from build123d import *

# Parameters (mm, degrees)
SKETCH_1_R          = 3.5
SKETCH_1_R_2        = 13
EXTRUDE_2_DEPTH     = 10
SKETCH_2_R          = 12.5
EXTRUDE_3_DEPTH     = 15
SKETCH_3_W          = 0.517195108
SKETCH_3_H          = 18.726193104
CUT_EXTRUDE_1_DEPTH = 26
SKETCH_4_R          = 2.5
CUT_EXTRUDE_2_DEPTH = 43.740275714


with BuildPart() as part:
    # 草图1 → 凸台-拉伸2 (new body)
    with BuildSketch(Plane.XY):
        with BuildLine():
            Line((-35, -7), (-7.740275714, -18.44147857))
            ThreePointArc((-7.740275714, -18.44147857), (0, -20), (7.740275714, -18.44147857))
            Line((7.740275714, -18.44147857), (35, -7))
            Line((35, -7), (35, 7))
            Line((35, 7), (7.740275714, 18.44147857))
            Line((7.740275714, 18.44147857), (7.740275714, 25.44147857))
            ThreePointArc((7.740275714, 25.44147857), (0, 27.494244152), (-7.740275714, 25.44147857))
            Line((-7.740275714, 25.44147857), (-7.740275714, 18.44147857))
            Line((-7.740275714, 18.44147857), (-35, 7))
            Line((-35, 7), (-35, -7))
        make_face()
        with Locations((-28, 0)):
            Circle(SKETCH_1_R, mode=Mode.SUBTRACT)
        Circle(SKETCH_1_R_2, mode=Mode.SUBTRACT)
        with Locations((28, 0)):
            Circle(SKETCH_1_R, mode=Mode.SUBTRACT)
    extrude(amount=EXTRUDE_2_DEPTH)

    # 草图2 → 凸台-拉伸3 (add)
    with BuildSketch(Plane.XY.offset(10)):
        with BuildLine():
            Line((-7.740275714, 18.44147857), (-7.740275714, 25.44147857))
            ThreePointArc((-7.740275714, 25.44147857), (0, 27.494244152), (7.740275714, 25.44147857))
            Line((7.740275714, 25.44147857), (7.740275714, 18.44147857))
            ThreePointArc((7.740275714, 18.44147857), (0, -20), (-7.740275714, 18.44147857))
        make_face()
        Circle(SKETCH_2_R, mode=Mode.SUBTRACT)
    extrude(amount=EXTRUDE_3_DEPTH)

    # 草图3 → 切除-拉伸1 (cut, through all)
    with BuildSketch(Plane.XY.offset(25)):
        with Locations((0, 21.741202931)):
            Rectangle(SKETCH_3_W, SKETCH_3_H)
    extrude(amount=-CUT_EXTRUDE_1_DEPTH, mode=Mode.SUBTRACT)

    # 草图4 → 切除-拉伸2 (cut, through all)
    with BuildSketch(Plane(origin=(7.740275714, 0, 0), x_dir=(0, 0, -1), z_dir=(1, 0, 0))):
        with Locations((-12.5, 21.086423576)):
            Circle(SKETCH_4_R)
    extrude(amount=-CUT_EXTRUDE_2_DEPTH, mode=Mode.SUBTRACT)


solid = part.part
Geometry: final body of the model. Coordinates: model frame, mm. A direction names the side the tool comes from. Give positions to 0.01 mm unless a question says otherwise; leave off trailing zeros. Loops run counter-clockwise (first coordinate to the right, second up) from the corner with the lowest first, then second, coordinate; pieces in that order, holes last. Notation, with made-up numbers: (-16, -16) - (32, -16) arc R25 ccw to (32, 18) - close; hole circle Ø8 at (42.5, 78.5). An arc over 180 degrees is marked (long way). One line per question, with ' | ' between items. Start each with the question number.
(1) Section query B-B on z = 7. Return loops of the section in (x, y).
(2) Section query A-A on x = 2. Return loops of the section in (y, z), then the cut area to 3 significant figures.
(3) Section query D-D on z = 18.25. Return loops of the section in (x, y).
(4) Reachability of faces 4 (the flat face through (7.74, 24, 12)), 5 (the flat face through (-7.74, 24, 12)), 6 (the flat face through (0.259, 18, 13)), 7 (the flat face through (35, 0, 5)), 8 (the cylindrical face through (31.34, 1.05, 4.93)) from +Z, -Z, +X, -X, +Y, -Y: full face, straight path, thin tool, end or side. Return the list, or none.
(5) Pull-direction query (Z, two-part tool) for faces 1 (the cylindrical face through (-3.947, 19.565, 14.484)), 2 (the flat face through (10.7, 6.8, 10)), 3 (the flat face through (-0.259, 18, 13)); classes: released by +Z, released by -Z, zero draft, split by the parting line, or undercut.
(6) Section query C-C on x = -11. Return loops of the section in (y, z).
(7) Ray query, line 1 (X direction, y = 22, z = 5); line 2 (Y direction, x = 5.5, z = 12.5); line 3 (Y direction, x = -3, z = 12.5). Return the intervals inside material, ascending. Write a range as from..to.
(8) Contact query for flat-ended pins moving along their axis: pin 1 (3.5 mm diameter, centred on y = 21, z = 8.5, fed in from +X); pin 2 (7.5 mm diameter, centred on y = 20.5, z = 12, fed in from -X); pin 3 (12 mm diameter, centred on y = 23, z = 6.5, fed in from -X). Output: stop coordinate, or through.
The answers:
1) outline: (-35, -7) - (-7.74, -18.44) arc R20 ccw to (7.74, -18.44) - (35, -7) - (35, 7) - (7.74, 18.44) - (7.74, 25.44) arc R15.62 ccw to (0.26, 27.49) - (0.26, 13) arc R13 cw (long way) to (-0.26, 13) - (-0.26, 27.49) arc R15.62 ccw to (-7.74, 25.44) - (-7.74, 18.44) - (-35, 7) - close; hole circle Ø7 at (-28, 0); hole circle Ø7 at (28, 0)
2) outline: (-19.9, 0) - (-12.85, 0) - (-12.85, 10) - (-12.34, 10) - (-12.34, 25) - (-19.9, 25) - close; (12.34, 10) - (12.85, 10) - (12.85, 0) - (27.37, 0) - (27.37, 25) - (12.34, 25) - close; hole circle Ø5 at (21.09, 12.5) | area: 535 mm2
3) outline: (-7.74, 18.44) arc R20 ccw (long way) to (7.74, 18.44) - (7.74, 25.44) arc R15.62 ccw to (0.26, 27.49) - (0.26, 12.5) arc R12.5 cw (long way) to (-0.26, 12.5) - (-0.26, 27.49) arc R15.62 ccw to (-7.74, 25.44) - close
4) face 4: +Z, -Z, +X, +Y | face 5: +Z, -Z, -X, +Y | face 6: +Z, -Z, +Y | face 7: +Z, -Z, +X, +Y, -Y | face 8: +Z, -Z
5) face 1: undercut | face 2: released by -Z | face 3: zero draft
6) outline: (-17.07, 0) - (-6.93, 0) - (-6.93, 10) - (-5.94, 10) - (-5.94, 25) - (-16.7, 25) - (-16.7, 10) - (-17.07, 10) - close; (5.94, 10) - (6.93, 10) - (6.93, 0) - (17.07, 0) - (17.07, 10) - (16.7, 10) - (16.7, 25) - (5.94, 25) - close
7) line 1: -7.74..-0.26, 0.26..7.74 | line 2: -19.23..-11.22, 11.22..18.59, 23.59..26.49 | line 3: -19.77..-12.13, 12.13..18.59, 23.59..27.2
8) pin 1: x = 7.74 | pin 2: x = -10.93 | pin 3: x = -11.17
